Can you work these out from the model? Positions are in its coordinate system, mm. Face numbers are marked on the shaded views. A direction names the side the tool comes from. Give positions to 0.01 mm unless a question says otherwise; leave off trailing zeros. Loops run counter-clockwise (first coordinate to the right, second up) from the corner with the lowest first, then second, coordinate; pieces in that order, holes last. Notation, with made-up numbers: M -31.5,18 L -11.5,18 A24 cw -11.5,38 Z; hole C 34.25,39 d9. An arc over 180 degrees is marked long. Answer as a JSON object with one key per item and string values.
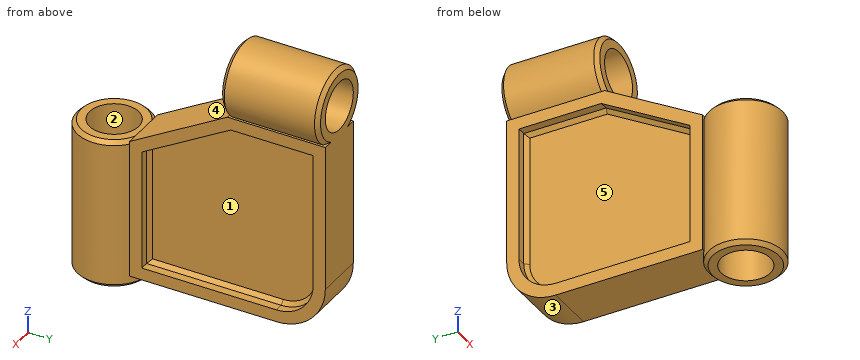
```python
from build123d import *

# Parameters (mm, degrees)
BOSS_EXTRUDE1_DEPTH      = 6.35
FILLET1_R                = 12.7
CUT_EXTRUDE2_DEPTH       = 3.175
BOSS_EXTRUDE2_DEPTH      = 3.175
BOSS_EXTRUDE2_DEPTH_BACK = 36.135303
SKETCH4_R                = 9.525
SKETCH4_R_2              = 6.35
SKETCH5_R                = 9.525
SKETCH5_R_2              = 6.35
BOSS_EXTRUDE3_DEPTH      = 25.4
CHAMFER2_SIZE            = 1
CHAMFER4_SIZE            = 1


with BuildPart() as part:
    # Sketch1 → Boss-Extrude1 (new, symmetric)
    with BuildSketch(Plane.YZ):
        Polygon((-25.4, 10.735303163), (0, 25.4), (25.4, 25.4), (25.4, -25.4), (-25.4, -25.4), align=None)
    extrude(amount=BOSS_EXTRUDE1_DEPTH, both=True)

    # Fillet1
    fillet1_edges = [part.edges().sort_by_distance(p)[0] for p in [
        (0, 25.4, -25.4),
    ]]
    fillet(fillet1_edges, radius=FILLET1_R)

    # Sketch3 → Cut-Extrude2 (cut)
    with BuildSketch(Plane.YZ.offset(6.35)):
        with BuildLine():
            Line((-22.225, -22.225), (12.7, -22.225))
            ThreePointArc((12.7, -22.225), (19.435192091, -19.435192091), (22.225, -12.7))
            Line((22.225, -12.7), (22.225, 22.225))
            Line((22.225, 22.225), (0.850738686, 22.225))
            Line((0.850738686, 22.225), (-22.225, 8.902216058))
            Line((-22.225, 8.902216058), (-22.225, -22.225))
        make_face()
    cut_extrude2 = extrude(amount=-CUT_EXTRUDE2_DEPTH, mode=Mode.SUBTRACT)

    # Mirror1: Cut-Extrude2 across plane
    add(cut_extrude2.mirror(Plane(origin=(0, 0, 0), x_dir=(0, 0, 1), z_dir=(1, 0, 0))), mode=Mode.SUBTRACT)

    # Sketch4 → Boss-Extrude2 (add, two sides: drawn at the far end of the back side and taken through both)
    with BuildSketch(Plane(origin=(0, 0, -25.4), x_dir=(1, 0, 0), z_dir=(0, 0, -1)).offset(-BOSS_EXTRUDE2_DEPTH_BACK)):
        with Locations(Location((0, 33.02, 0), (0, 0, 233.130102354))):
            Circle(SKETCH4_R)
        with Locations(Location((0, 33.02, 0), (0, 0, 270))):
            Circle(SKETCH4_R_2, mode=Mode.SUBTRACT)
    extrude(amount=BOSS_EXTRUDE2_DEPTH + BOSS_EXTRUDE2_DEPTH_BACK)

    # Sketch5 → Boss-Extrude3 (add)
    with BuildSketch(Plane(origin=(0, 25.4, 0), x_dir=(-1, 0, 0), z_dir=(0, 1, 0))):
        with Locations((0, 33.02)):
            Circle(SKETCH5_R)
        with Locations(Location((0, 33.02, 0), (0, 0, 90))):
            Circle(SKETCH5_R_2, mode=Mode.SUBTRACT)
    extrude(amount=-BOSS_EXTRUDE3_DEPTH)

    # Chamfer2
    # the kernel refuses this chamfer: 1 mm, written as the material it takes off along each edge
    with BuildSketch(Plane(origin=(0, -33.02, 10.735303), x_dir=(0.3638595085405839, 0.931453841070294, 0), z_dir=(-0.931453841070294, 0.3638595085405839, 0))) as chamfer2_piece_1_section:
        Polygon((9.525, CHAMFER2_SIZE), (9.525 - CHAMFER2_SIZE, 0), (9.525, 0), align=None)
    chamfer2_piece_1 = revolve(axis=Axis((0, -33.02, 10.735303), (0, 0, -1)), revolution_arc=317.325176487, mode=Mode.PRIVATE)
    chamfer2_piece_1 = split(chamfer2_piece_1, bisect_by=Plane(origin=(5.777045626, -25.4, 10.24862198), z_dir=(0, -1, 0)), keep=Keep.TOP, mode=Mode.PRIVATE)
    add(chamfer2_piece_1, mode=Mode.SUBTRACT)
    with BuildSketch(Plane(origin=(0, -33.02, -28.575), x_dir=(-0.6000000000021781, 0.7999999999983665, 0), z_dir=(-0.7999999999983665, -0.6000000000021781, 0))) as chamfer2_piece_2:
        Polygon((9.525, -CHAMFER2_SIZE), (9.525 - CHAMFER2_SIZE, 0), (9.525, 0), align=None)
    revolve(axis=Axis((0, -33.02, -28.575), (0, 0, -1)), mode=Mode.SUBTRACT)
    with BuildSketch(Plane(origin=(0, 25.4, 33.02), x_dir=(-0.3638595085405501, 0, -0.9314538410703074), z_dir=(0.9314538410703074, 0, -0.3638595085405501))) as chamfer2_piece_3_section:
        Polygon((9.525, -CHAMFER2_SIZE), (9.525 - CHAMFER2_SIZE, 0), (9.525, 0), align=None)
    chamfer2_piece_3 = revolve(axis=Axis((0, 25.4, 33.02), (0, 1, 0)), revolution_arc=317.325176487, mode=Mode.PRIVATE)
    chamfer2_piece_3 = split(chamfer2_piece_3, bisect_by=Plane(origin=(0, 24.920234358, 25.4), z_dir=(0, 0, 1)), keep=Keep.TOP, mode=Mode.PRIVATE)
    add(chamfer2_piece_3, mode=Mode.SUBTRACT)
    with BuildSketch(Plane(origin=(0, 0, 33.02), x_dir=(-0.3638595085405531, 0, -0.9314538410703063), z_dir=(0.9314538410703063, 0, -0.3638595085405531))) as chamfer2_piece_4_section:
        Polygon((9.525, CHAMFER2_SIZE), (9.525 - CHAMFER2_SIZE, 0), (9.525, 0), align=None)
    chamfer2_piece_4 = revolve(axis=Axis((0, 0, 33.02), (0, 1, 0)), revolution_arc=317.325176487, mode=Mode.PRIVATE)
    chamfer2_piece_4 = split(chamfer2_piece_4, bisect_by=Plane(origin=(-5.452412952, 0.490850729, 25.4), z_dir=(0, 0, 1)), keep=Keep.TOP, mode=Mode.PRIVATE)
    add(chamfer2_piece_4, mode=Mode.SUBTRACT)

    # Chamfer4
    chamfer4_edges = [part.edges().sort_by_distance(p)[0] for p in [
        (3.175, -22.225, -6.661391971),
        (3.175, -10.687130657, 15.563608029),
        (3.175, 11.537869343, 22.225),
        (3.175, 22.225, 4.7625),
        (3.175, 19.435192091, -19.435192091),
        (3.175, -4.7625, -22.225),
        (-3.175, -22.225, -6.661391971),
        (-3.175, -4.7625, -22.225),
        (-3.175, 19.435192091, -19.435192091),
        (-3.175, 22.225, 4.7625),
        (-3.175, 11.537869343, 22.225),
        (-3.175, -10.687130657, 15.563608029),
    ]]
    chamfer(chamfer4_edges, length=CHAMFER4_SIZE)


solid = part.part
```
1) Please list where these lines run through material, in increasing order: line 1 along X through (y, z) = (8, 33); line 2 along Y through (x, z) = (-0.5, 9); line 3 along Z through (x, y) = (3.75, 14.5). Write a range as from..to.
Answer list:
{"line 1": "-9.52..-6.35, 6.35..9.52", "line 2": "-42.53..-39.35, -26.69..25.4", "line 3": "-25.27..-21.62, 21.8..27.9, 38.14..41.78"}
2) For the marked faces 1 and 2, which set-ups out of +Z, -Z, +X, -X, +Y, -Y let a thin tool reach every point of the face, with its end or its side?
Answer list:
{"face 1": "+X", "face 2": "+Z, -Z"}
3) Suppose I cut it at D-D, the plane y = 8. Write out the boundary of the cut face in (x, z) (3 decimals), and give its area (3 significant figures).
Answer list:
{"outline": "M -6.35,-25.4 L 6.35,-25.4 L 6.35,-22.225 L 4.175,-22.225 L 3.175,-21.225 L 3.175,21.225 L 4.175,22.225 L 6.35,22.225 L 6.35,25.4 L 5.715,25.4 A9.525 ccw long -5.715,25.4 L -6.35,25.4 L -6.35,22.225 L -4.175,22.225 L -3.175,21.225 L -3.175,-21.225 L -4.175,-22.225 L -6.35,-22.225 Z; hole C 0,33.02 d12.7", "area": "508 mm^2"}
4) Suppose I cut it at C-C, the plane x = 0. Write out the boundary of the cut face in (y, z) (3 decimals), and give its area (3 significant figures).
Answer list:
{"outline": "M -42.545,-27.575 L -41.545,-28.575 L -39.37,-28.575 L -39.37,10.735 L -41.545,10.735 L -42.545,9.735 Z; M -26.67,-28.575 L -24.495,-28.575 L -23.495,-27.575 L -23.495,-25.4 L 12.7,-25.4 A12.7 ccw 25.4,-12.7 L 25.4,26.67 L 0,26.67 L 0,25.4 L -25.4,10.735 L -26.67,10.735 Z; M 0,39.37 L 25.4,39.37 L 25.4,41.545 L 24.4,42.545 L 1,42.545 L 0,41.545 Z", "area": "2,650 mm^2"}
5) Suppose I cut it at B-B, the plane y = -33.02. Write out the boundary of the cut face in (x, z) (3 decimals), and give its area (3 significant figures).
Answer list:
{"outline": "M -9.525,-27.575 L -8.525,-28.575 L -6.35,-28.575 L -6.35,10.735 L -8.525,10.735 L -9.525,9.735 Z; M 6.35,-28.575 L 8.525,-28.575 L 9.525,-27.575 L 9.525,9.735 L 8.525,10.735 L 6.35,10.735 Z", "area": "248 mm^2"}
6) Suppose I cut it at A-A, the plane z = 33.02. Write out the boundary of the cut face in (x, y) (3 decimals).
Answer list:
{"outline": "M -9.525,1 L -8.525,0 L -6.35,0 L -6.35,25.4 L -8.525,25.4 L -9.525,24.4 Z; M 6.35,0 L 8.525,0 L 9.525,1 L 9.525,24.4 L 8.525,25.4 L 6.35,25.4 Z"}
7) Will these pins go through, and if not, where does the flat tip stop? pin 1 Ø4 at (x, y) = (7, -13) entering from +Z; pin 2 Ø0.7 at (x, y) = (-5.5, 10) entering from -Z; pin 3 Ø1.1 at (x, z) = (-5.5, -3) entering from -Y.
Answer list:
{"pin 1": "z = 18.99", "pin 2": "z = -25.4", "pin 3": "y = -41.16"}
8) If we mould it in two halves opening along Z, with no side actions, what happens to the marked faces 3, 4 and 5? For each: +Z half, -Z half, draft (parallel to the pull), parting line (faces both ways), or undercut.
Answer list:
{"face 3": "-Z half", "face 4": "+Z half", "face 5": "undercut"}
